Geometry: see drawing. Coordinates: mm, zero at the bounding-box minimum. A direction names the side the tool comes from. Coordinates: 2 decimals unless noted, no trailing zeros. Loops run counter-clockwise (first coordinate to the right, second up) from the corner with the lowest first, then second, coordinate; pieces in that order, holes last. Notation, with made-up numbers: (63.5, -40) - (104.5, -40) arc R14 ccw to (104.5, -26) - close; hole circle Ø2 at (13, 61.25). An arc over 180 degrees is marked (long way). Answer in a Markdown table with one row per item.
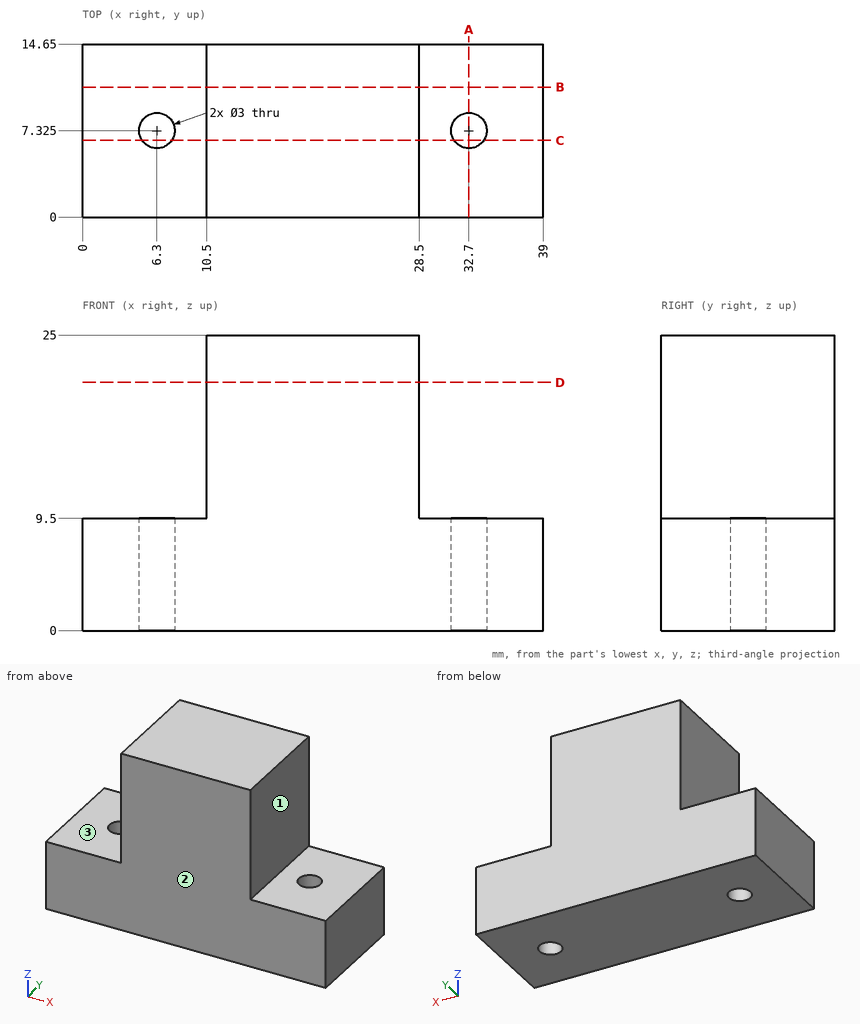
(1) Cut plane D-D on z = 21. Output: boundary loops of the cut face in (x, y).
Verdict:
| item | result |
|---|---|
| outline | (10.5, 0) - (28.5, 0) - (28.5, 14.65) - (10.5, 14.65) - close |
(2) Cut plane A-A on x = 32.7. Output: boundary loops of the cut face in (y, z) (3 decimals), then the cut area to 3 significant figures.
Verdict:
| item | result |
|---|---|
| outline | (0, 0) - (5.825, 0) - (5.825, 9.5) - (0, 9.5) - close; (8.825, 0) - (14.65, 0) - (14.65, 9.5) - (8.825, 9.5) - close |
| area | 111 mm² |
(3) First-contact query: pin 1 Ø6 at (x, y) = (9, 11) entering from +Z; pin 2 Ø7.5 at (y, z) = (4, 19.5) entering from -X; pin 3 Ø4.5 at (y, z) = (5, 19) entering from +X; pin 4 Ø3 at (x, y) = (35, 7) entering from +Z. Flat tips, straight axial feed; report the tip coordinate or a pass-through.
Verdict:
| item | result |
|---|---|
| pin 1 | stops at z = 25 |
| pin 2 | stops at x = 10.5 |
| pin 3 | stops at x = 28.5 |
| pin 4 | stops at z = 9.5 |
(4) Access query for the marked faces 1, 2 and 3. Directions: +Z, -Z, +X, -X, +Y, -Y. A direction counts if a zero-diameter tool reaches every point of the face in a straight line with its end or side. Return the directions, or none.
Verdict:
| item | result |
|---|---|
| face 1 | +Z, +X, +Y, -Y |
| face 2 | +Z, -Z, +X, -X, -Y |
| face 3 | +Z, -X, +Y, -Y |
(5) Cut plane C-C on y = 6.5. Output: boundary loops of the cut face in (x, z).
Verdict:
| item | result |
|---|---|
| outline | (0, 0) - (5.05, 0) - (5.05, 9.5) - (0, 9.5) - close; (7.55, 0) - (31.45, 0) - (31.45, 9.5) - (28.5, 9.5) - (28.5, 25) - (10.5, 25) - (10.5, 9.5) - (7.55, 9.5) - close; (33.95, 0) - (39, 0) - (39, 9.5) - (33.95, 9.5) - close |
(6) Ray query, probe 1 along Y at (x, z) = (32.7, 6.5) (3 decimals); probe 2 along Z at (x, y) = (5.5, 4.75); probe 3 along X at (y, z) = (5.5, 16). Return the intervals inside material, ascending.
Verdict:
| item | result |
|---|---|
| probe 1 | y = 0 to 5.825, 8.825 to 14.65 |
| probe 2 | z = 0 to 9.5 |
| probe 3 | x = 10.5 to 28.5 |
(7) Cut plane B-B on y = 11. Output: boundary loops of the cut face in (x, z), then the cut area to 4 significant figures.
Verdict:
| item | result |
|---|---|
| outline | (0, 0) - (39, 0) - (39, 9.5) - (28.5, 9.5) - (28.5, 25) - (10.5, 25) - (10.5, 9.5) - (0, 9.5) - close |
| area | 649.5 mm² |
